Input: part model. Units: mm. Frame: model coordinates. Face numbers are marked on the shaded views. Give positions to 0.01 mm unless a question says otherwise; leave off trailing zeros. Loops run counter-clockwise (first coordinate to the right, second up) from the corner with the lowest first, then second, coordinate; pieces in that order, holes last. Notation, with made-up numbers: M 7,21 L 16,21 A19 ccw 16,38 Z; hole C -30,-22 d1. An arc over 180 degrees is marked long. One line per item, written item: value. Start each with the question number.
(1) Section B-B on x = 6.35. Output: boundary loops of the cut face in (y, z), plus the area to 3 significant figures.
(2) Ray query, line 1 along X through (y, z) = (5.25, -12.7); line 2 along X through (y, z) = (3.25, -6.35); line 3 along Z through (x, y) = (12.7, 2.5). Return the intervals inside material, ascending. Write a range as from..to.
(3) Pull-direction query (Z, two-part tool) for the marked faces 1, 2 and 3; classes: released by +Z, released by -Z, zero draft, split by the parting line, or undercut.
(4) Section A-A on z = 0. Output: boundary loops of the cut face in (x, y) (3 decimals).
(5) Section C-C on y = 3. State how many separate pieces and enclosed holes the cut face has, plus the area to 3 significant figures.
```python
from build123d import *

# Parameters (mm, degrees)
SKETCH1_W           = 38.1
SKETCH1_H           = 38.1
SKETCH1_R           = 1.778
SKETCH1_R_2         = 1.7907
SKETCH1_R_3         = 1.8034
SKETCH1_R_4         = 1.8161
SKETCH1_R_5         = 1.8288
SKETCH1_R_6         = 1.8542
SKETCH1_R_7         = 1.8669
SKETCH1_R_8         = 1.8796
SKETCH1_R_9         = 1.8923
SKETCH1_R_10        = 1.9177
SKETCH1_R_11        = 1.9304
SKETCH1_R_12        = 1.9431
SKETCH1_R_13        = 1.9558
SKETCH1_R_14        = 1.9812
SKETCH1_R_15        = 1.9939
SKETCH1_R_16        = 2.0066
SKETCH1_R_17        = 2.0193
SKETCH1_R_18        = 2.0447
SKETCH1_R_19        = 2.0574
SKETCH1_R_20        = 2.0701
SKETCH1_R_21        = 2.0828
SKETCH1_R_22        = 1.8415
SKETCH1_R_23        = 1.905
SKETCH1_R_24        = 1.9685
SKETCH1_R_25        = 2.032
BOSS_EXTRUDE1_DEPTH = 6.35


with BuildPart() as part:
    # Sketch1 → Boss-Extrude1 (new body)
    with BuildSketch(Plane(origin=(0, 0, 0), x_dir=(1, 0, 0), z_dir=(0, 1, 0))):
        Rectangle(SKETCH1_W, SKETCH1_H)
        with Locations((-12.7, 12.7)):
            Circle(SKETCH1_R, mode=Mode.SUBTRACT)
        with Locations((-6.35, 12.7)):
            Circle(SKETCH1_R_2, mode=Mode.SUBTRACT)
        with Locations((0, 12.7)):
            Circle(SKETCH1_R_3, mode=Mode.SUBTRACT)
        with Locations((6.35, 12.7)):
            Circle(SKETCH1_R_4, mode=Mode.SUBTRACT)
        with Locations((12.7, 12.7)):
            Circle(SKETCH1_R_5, mode=Mode.SUBTRACT)
        with Locations((-6.35, 6.35)):
            Circle(SKETCH1_R_6, mode=Mode.SUBTRACT)
        with Locations((0, 6.35)):
            Circle(SKETCH1_R_7, mode=Mode.SUBTRACT)
        with Locations((6.35, 6.35)):
            Circle(SKETCH1_R_8, mode=Mode.SUBTRACT)
        with Locations((12.7, 6.35)):
            Circle(SKETCH1_R_9, mode=Mode.SUBTRACT)
        with Locations((-6.35, 0)):
            Circle(SKETCH1_R_10, mode=Mode.SUBTRACT)
        Circle(SKETCH1_R_11, mode=Mode.SUBTRACT)
        with Locations((6.35, 0)):
            Circle(SKETCH1_R_12, mode=Mode.SUBTRACT)
        with Locations((12.7, 0)):
            Circle(SKETCH1_R_13, mode=Mode.SUBTRACT)
        with Locations((-6.35, -6.35)):
            Circle(SKETCH1_R_14, mode=Mode.SUBTRACT)
        with Locations((0, -6.35)):
            Circle(SKETCH1_R_15, mode=Mode.SUBTRACT)
        with Locations((6.35, -6.35)):
            Circle(SKETCH1_R_16, mode=Mode.SUBTRACT)
        with Locations((12.7, -6.35)):
            Circle(SKETCH1_R_17, mode=Mode.SUBTRACT)
        with Locations((-6.35, -12.7)):
            Circle(SKETCH1_R_18, mode=Mode.SUBTRACT)
        with Locations((0, -12.7)):
            Circle(SKETCH1_R_19, mode=Mode.SUBTRACT)
        with Locations((6.35, -12.7)):
            Circle(SKETCH1_R_20, mode=Mode.SUBTRACT)
        with Locations((12.7, -12.7)):
            Circle(SKETCH1_R_21, mode=Mode.SUBTRACT)
        with Locations((-12.7, 6.35)):
            Circle(SKETCH1_R_22, mode=Mode.SUBTRACT)
        with Locations((-12.7, 0)):
            Circle(SKETCH1_R_23, mode=Mode.SUBTRACT)
        with Locations((-12.7, -6.35)):
            Circle(SKETCH1_R_24, mode=Mode.SUBTRACT)
        with Locations((-12.7, -12.7)):
            Circle(SKETCH1_R_25, mode=Mode.SUBTRACT)
    extrude(amount=BOSS_EXTRUDE1_DEPTH)


solid = part.part
```
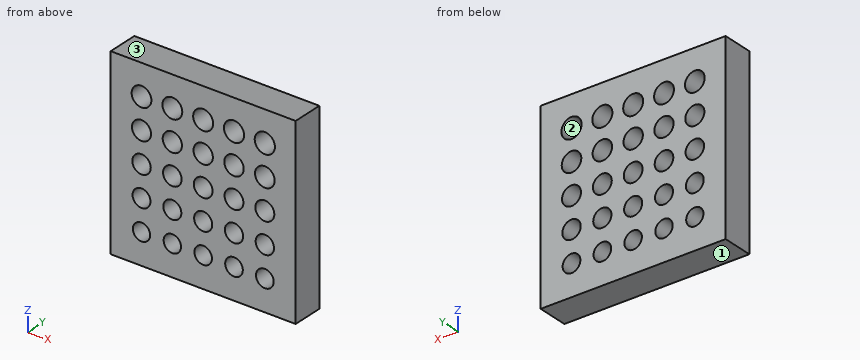
Output values:
1. outline: M 0,-19.05 L 6.35,-19.05 L 6.35,-14.52 L 0,-14.52 Z; M 0,-10.88 L 6.35,-10.88 L 6.35,-8.23 L 0,-8.23 Z; M 0,-4.47 L 6.35,-4.47 L 6.35,-1.94 L 0,-1.94 Z; M 0,1.94 L 6.35,1.94 L 6.35,4.34 L 0,4.34 Z; M 0,8.36 L 6.35,8.36 L 6.35,10.63 L 0,10.63 Z; M 0,14.77 L 6.35,14.77 L 6.35,19.05 L 0,19.05 Z
1. area: 119 mm²
2. line 1: x = -19.05..-14.48, -10.92..-8.14, -4.56..-1.8, 1.8..4.53, 8.17..10.87, 14.53..19.05
2. line 2: x = -19.05..-14.54, -10.86..-8.2, -4.5..-1.87, 1.87..4.47, 8.23..10.81, 14.59..19.05
2. line 3: z = -19.05..-14.53, -10.87..-8.24, -4.46..-1.96, 1.96..4.33, 8.37..10.62, 14.78..19.05
3. face 1: released by -Z
3. face 2: undercut
3. face 3: released by +Z
4. outline: M -19.05,0 L -14.605,0 L -14.605,6.35 L -19.05,6.35 Z; M -10.795,0 L -8.268,0 L -8.268,6.35 L -10.795,6.35 Z; M -4.432,0 L -1.93,0 L -1.93,6.35 L -4.432,6.35 Z; M 1.93,0 L 4.407,0 L 4.407,6.35 L 1.93,6.35 Z; M 8.293,0 L 10.744,0 L 10.744,6.35 L 8.293,6.35 Z; M 14.656,0 L 19.05,0 L 19.05,6.35 L 14.656,6.35 Z
5. separate pieces: 1
5. enclosed holes: 25
5. area: 1,160 mm²
